Answer from the drawing. Dimensions are ordinates in mm from the lowest x, y and z of the part. A direction names the side the tool comes from. Give positions to 0.01 mm unless a question says otherwise; leave off trailing zeros. Loops run counter-clockwise (first coordinate to the right, second up) from the corner with the lowest first, then second, coordinate; pieces in that order, holes last.
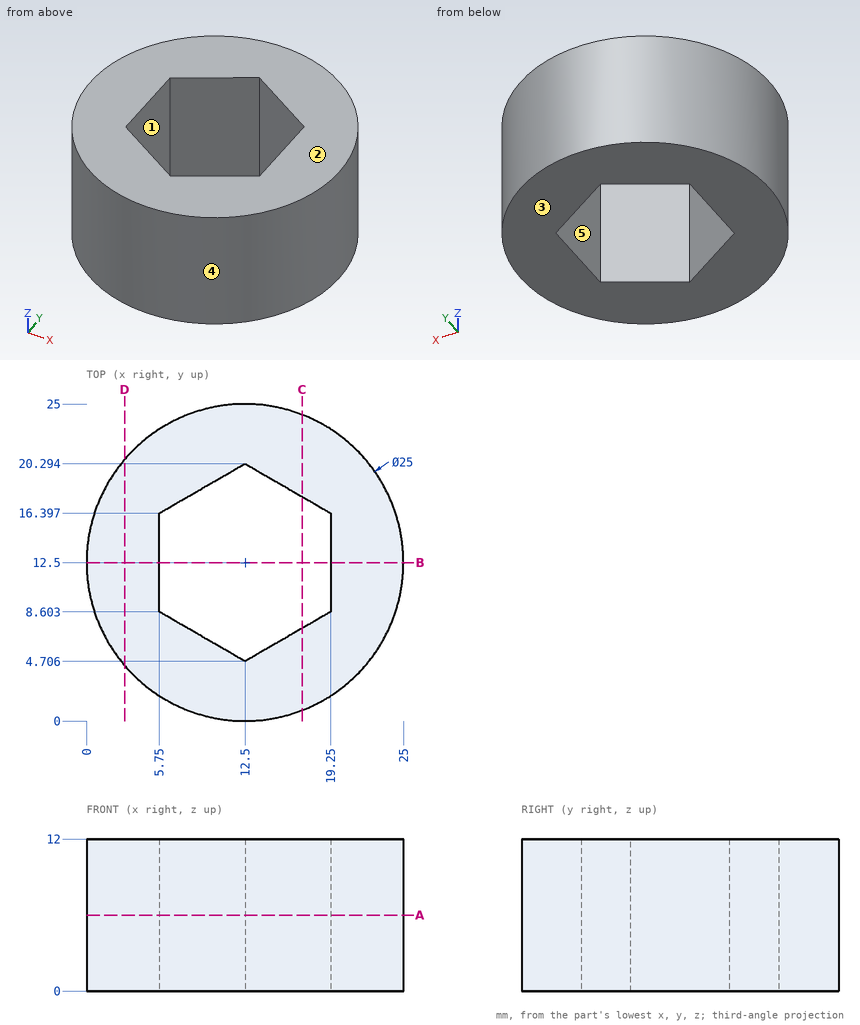
Item 1: Determine the mould class of the marked faces 3, 4 and 5 for opening direction X: released by +X, released by -X, zero draft, split by the parting line, or undercut.
Item 2: Flat-ended cylindrical pins translate along their axes: pin 1 Ø6 at (y, z) = (4.5, 8) entering from +X; pin 2 Ø5 at (x, z) = (17, 6) entering from +Y; pin 3 Ø4 at (x, z) = (20.5, 4) entering from -Y. Find the tip coordinate at first contact, or state that the pin passes through.
Item 3: Find section D-D, the plane x = 3. Write down the section's boundary in (y, z), plus the area to 3 significant figures.
Item 4: For the marked faces 1 and 2, determine the directions among +Z, -Z, +X, -X, +Y, -Y from which every point of the face is accessible in a straight line to the end or side of a thin tool.
Item 5: Find section C-C, the plane x = 17. Write down the section's boundary in (y, z).
Item 6: Consider line 1 (X direction, y = 8.5, z = 2.75); line 2 (Y direction, x = 15, z = 6.25); line 3 (Y direction, x = 7.25, z = 5) (1 decimal). Determine where each line is inside the solid, lowest interval first.
Item 7: Find section A-A, the plane z = 6. Write down the section's boundary in (x, y), plus the area to 3 significant figures.
Item 8: Find section B-B, the plane y = 12.5. Write down the section's boundary in (x, z).
Ans:
1. face 3: zero draft
1. face 4: split by the parting line
1. face 5: undercut
2. pin 1: stops at x = 23.96
2. pin 2: stops at y = 24.84
2. pin 3: stops at y = 1.53
3. outline: (4.38, 0) - (20.62, 0) - (20.62, 12) - (4.38, 12) - close
3. area: 195 mm2
4. face 1: +Z, -Z
4. face 2: +Z, +X, -X, +Y, -Y
5. outline: (0.84, 0) - (7.3, 0) - (7.3, 12) - (0.84, 12) - close; (17.7, 0) - (24.16, 0) - (24.16, 12) - (17.7, 12) - close
6. line 1: x = 0.66 to 5.93, 19.07 to 24.34
6. line 2: y = 0.25 to 6.15, 18.85 to 24.75
6. line 3: y = 1.2 to 7.7, 17.3 to 23.8
7. outline: circle Ø25 at (12.5, 12.5); hole (5.75, 8.6) - (12.5, 4.71) - (19.25, 8.6) - (19.25, 16.4) - (12.5, 20.29) - (5.75, 16.4) - close
7. area: 333 mm2
8. outline: (0, 0) - (5.75, 0) - (5.75, 12) - (0, 12) - close; (19.25, 0) - (25, 0) - (25, 12) - (19.25, 12) - close
